Design review of the part built by this model. Coordinates are the model's own, in mm. Face numbers are marked on the shaded views. A direction names the side the tool comes from. Coordinates: 2 decimals unless noted, no trailing zeros. Write each loop counter-clockwise with the first axis right and the second up, starting at its lowest first coordinate (ties: lowest second). Pieces come first, ordered by that corner, then holes. Notation, with made-up numbers: M 76.5,70.25 L 131.5,70.25 A27 cw 131.5,98.25 Z; hole C 78,6 d6. An arc over 180 degrees is marked long. Return JSON: item names as keys, results as strings. Group by question number.
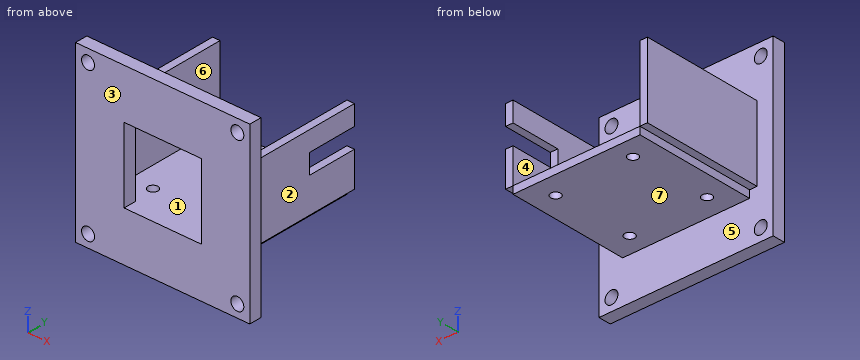
Autodesk Inventor part; units mm, degrees
ref_plane "YZ Plane" through (0, 0, 0) normal (1, 0, 0) x (0, 1, 0)
ref_plane "XZ Plane" through (0, 0, 0) normal (0, 1, 0) x (-1, 0, 0)
ref_plane "XY Plane" through (0, 0, 0) normal (0, 0, 1) x (1, 0, 0)
sketch "Boceto1" plane through (0, 0, 0) normal (0, 1, 0) x (-1, 0, 0)
  line L0 (25.5, 15) -> (-25.5, 15)
  line L1 (-25.5, 15) -> (-25.5, -15)
  line L2 (-25.5, -15) -> (25.5, -15)
  line L3 (25.5, -15) -> (25.5, 15)
  line L4 (25.5, 15) -> (-25.5, -15) construction
  line L5 (-25.5, 15) -> (25.5, -15) construction
  line L6 (-15.5, 15) -> (-15.5, -15)
  line L7 (0, 15) -> (0, 11.847)
  line L8 (-25.5, 0) -> (-22.3332, 0)
  line L9 (25.5, 15) -> (25.5, -15)
  line L10 (15.5, 15) -> (15.5, -15)
  line L11 (25.5, 0) -> (22.3332, 0)
  line L12 (-25.5, -15) -> (-25.5, 15)
  line L13 (-25.5, 0) -> (-22.3332, 0)
  line L14 (-25.5, 15) -> (-25.5, -15)
  point P0 (0, 0)
  point P1 (31.5, 22.5)
  dimension "d2" = 10
  dimension "d21" = 51
  dimension "d22" = 30
extrude "Extrusión1" add sketch "Boceto1" along normal blind 5 contours L3 L2 L10 L0 | L6 L2 L1 L0
sketch "Boceto4" plane through (0, 0, 0) normal (0, 1, 0) x (-1, 0, 0)
  line L0 (-28.5, 18) -> (28.5, 18)
  line L1 (28.5, 18) -> (28.5, -18)
  line L2 (28.5, -18) -> (-28.5, -18)
  line L3 (-28.5, -18) -> (-28.5, 18)
  line L4 (-28.5, 18) -> (28.5, -18) construction
  line L5 (28.5, 18) -> (-28.5, -18) construction
  line L6 (28.5, -15) -> (-28.5, -15)
  line L7 (-28.5, 15) -> (28.5, 15)
  line L8 (25.5, -18) -> (25.5, 18)
  line L9 (-25.5, 18) -> (-25.5, -18)
  line L10 (-25.5, -15) -> (-15.5, -15)
  point P0 (0, 0)
  point P1 (-25.5, -15)
  point P2 (-25.5, 15)
  point P3 (25.5, 15)
  point P4 (25.5, -15)
  dimension "d23" = 57
  dimension "d24" = 36
  dimension "d27" = 0
extrude "Extrusión4" add sketch "Boceto4" along normal blind 5 contours L0 L8 L7 L9 | L7 L9 L6 L3 | L7 L1 L6 L8 | L6 L8 L2 L9
sketch "Boceto5" plane through (0, 5, 0) normal (0, 1, 0) x (1, 0, 0)
  line L0 (25.5, 18) -> (-25.5, 18)
  line L1 (25.5, 15) -> (25.5, 18)
  line L2 (-25.5, 18) -> (25.5, 18)
  line L3 (25.5, 18) -> (25.5, 15)
  line L4 (25.5, 15) -> (-25.5, 15)
  line L5 (-25.5, 15) -> (-25.5, 18)
  point P0 (0, 0)
extrude "Extrusión5" add sketch "Boceto5" along normal blind 49
sketch "Boceto6" plane through (-15.5, 0, -15) normal (0, 0, 1) x (1, 0, 0)
  circle A0 centre (32, 45) radius 2
  line L0 (41, 5) -> (41, 54)
  line L1 (-10, 54) -> (41, 54)
  line L2 (-10, 5) -> (-10, 54)
  line L3 (-10, 29.5) -> (15.5, 29.5)
  line L4 (15.5, 29.5) -> (15.5, 54)
  circle A1 centre (0, 46) radius 2
  circle A2 centre (-1, 14) radius 2
  circle A3 centre (31, 13) radius 2
  point P0 (15.5, 0)
  dimension "d30" = 4
  dimension "d31" = 9
  dimension "d32" = 9
  dimension "d35" = 360
extrude "Extrusión6" cut sketch "Boceto6" against normal blind 49 contours A0 | A1 | A2 | A3
sketch "Boceto7" plane through (0, 5, 0) normal (0, 1, 0) x (1, 0, 0)
  line L0 (-28.5, 15) -> (-28.5, -15)
  line L1 (-28.5, 15) -> (-25.5, 15)
  line L2 (-25.5, 15) -> (-25.5, -15)
  line L3 (-25.5, -15) -> (-28.5, -15)
  line L4 (-28.5, -15) -> (-28.5, 15)
  line L5 (28.5, 15) -> (25.5, 15)
  line L6 (25.5, -15) -> (28.5, -15)
  line L7 (28.5, 15) -> (25.5, 15)
  line L8 (25.5, 15) -> (25.5, -15)
  line L9 (25.5, -15) -> (28.5, -15)
  line L10 (28.5, -15) -> (28.5, 15)
  point P0 (0, 0)
  point P1 (25.5, -18)
extrude "Extrusión7" add sketch "Boceto7" along normal blind 49
sketch "Boceto12" plane through (0, 0, 0) normal (0, -1, 0) x (1, 0, 0)
  line L0 (-35, -35) -> (35, -35)
  line L1 (35, -35) -> (35, 35)
  line L2 (35, 35) -> (-35, 35)
  line L3 (-35, 35) -> (-35, -35)
  line L4 (-35, -35) -> (35, 35) construction
  line L5 (35, -35) -> (-35, 35) construction
  line L6 (30, 30) -> (-30, 30)
  line L7 (-30, 30) -> (-30, -30)
  line L8 (-30, -30) -> (30, -30)
  line L9 (30, -30) -> (30, 30)
  line L10 (30, 30) -> (-30, -30) construction
  line L11 (-30, 30) -> (30, -30) construction
  circle A0 centre (-30, 30) radius 2.6
  circle A1 centre (30, 30) radius 2.6
  circle A2 centre (30, -30) radius 2.6
  circle A3 centre (-30, -30) radius 2.6
  line L12 (15.5, -15) -> (15.5, 15)
  line L13 (-15.5, -15) -> (15.5, -15)
  line L14 (15.5, -15) -> (15.5, 15)
  line L15 (15.5, 15) -> (-15.5, 15)
  line L16 (-15.5, 15) -> (-15.5, -15)
  line L17 (-15.5, -15) -> (15.5, 15) construction
  line L18 (15.5, -15) -> (-15.5, 15) construction
  point P0 (0, 0)
  point P1 (0, 0)
  dimension "d63" = 70
  dimension "d64" = 70
  dimension "d65" = 60
  dimension "d66" = 5.2
  dimension "d67" = 5.2
  dimension "d68" = 5.2
  dimension "d69" = 5.2
extrude "Extrusión10" add sketch "Boceto12" against normal blind 5 contours L3 L2 L1 L0 | L6 A1 L9 A2 L8 A3 L7 A0
sketch "Boceto13" plane through (28.5, 5, 15) normal (1, 0, 0) x (0, 0, -1)
  line L0 (0, 49) -> (30, 49)
  line L1 (8, 49) -> (16, 49)
  line L2 (16, 49) -> (16, 29)
  line L3 (16, 29) -> (8, 29)
  line L4 (8, 29) -> (8, 49)
  line L5 (0, 0) -> (0, 49)
  point P0 (15, -5)
  dimension "d72" = 8
  dimension "d73" = 20
  dimension "d74" = 8
extrude "Extrusión11" cut sketch "Boceto13" against normal blind 10
properties part number "short-depth"
Item 1: For line 1 (Z direction, x = -30, y = 1.15); line 2 (Y direction, x = -16.5, z = -15.8); line 3 (Z direction, x = 12, y = 48), list the stretches that pass through material, from the lowest coordinate up.
Item 2: Add section A-A (z = 30). Write out the cut boundary in (x, y).
Item 3: For pin 1 (0.9 mm diameter, centred on y = 36.5, z = -16, fed in from +X); pin 2 (3 mm diameter, centred on x = -16.5, y = 14, fed in from -Z); pin 3 (1.5 mm diameter, centred on x = 27.5, y = 37, fed in from -Z); pin 4 (12 mm diameter, centred on x = -16.5, y = 39.5, fed in from +Z), all flat-tipped, find the tip position at first contact; note any pin that passes through.
Item 4: The part is to be moulded in two halves that separate along X. For the marked faces 1, 2, 3 and 4, say which applies: pulls with the +X half, pulls with the -X half, needs draft (parallel to the pull), parting line crosses it, or undercut.
Item 5: Machinability: for the marked faces 5, 6 and 7, which of the approach directions +Z, -Z, +X, -X, +Y, -Y give a long, thin tool a straight path to every point of the face, cutting with its end or side? Answer none if there is none.
Item 6: Add section C-C (x = 9.5). Write out the cut boundary in (y, z), plus the area to 3 significant figures.
Item 7: Add section D-D (z = 12.5). Write out the cut boundary in (x, y).
Geometry check:
{
 "1": {"line 1": "-35 to -32.6, -27.4 to 27.4, 32.6 to 35", "line 2": "0 to 12, 16 to 44.27, 47.73 to 54", "line 3": "-18 to -15"},
 "2": {"outline": "M -35,0 L -32.6,0 L -32.6,5 L -35,5 Z; M -27.4,0 L 27.4,0 L 27.4,5 L -27.4,5 Z; M 32.6,0 L 35,0 L 35,5 L 32.6,5 Z"},
 "3": {"pin 1": "x = 25.5", "pin 2": "through", "pin 3": "z = -15", "pin 4": "z = -15"},
 "4": {"face 1": "undercut", "face 2": "pulls with the +X half", "face 3": "needs draft", "face 4": "undercut"},
 "5": {"face 5": "+Y", "face 6": "+Z, +Y", "face 7": "-Z, +X, -X, +Y"},
 "6": {"outline": "M 0,-35 L 5,-35 L 5,-18 L 54,-18 L 54,-15 L 0,-15 Z; M 0,15 L 5,15 L 5,35 L 0,35 Z", "area": "347 mm^2"},
 "7": {"outline": "M -35,0 L -15.5,0 L -15.5,5 L -25.5,5 L -25.5,54 L -28.5,54 L -28.5,5 L -35,5 Z; M 15.5,0 L 35,0 L 35,5 L 28.5,5 L 28.5,54 L 25.5,54 L 25.5,5 L 15.5,5 Z"}
}
